```python
from build123d import *

# Parameters (mm, degrees)
CORTE_EXTRUS_O3_REACH         = 46.677
RESSALTO_EXTRUS_O1_DEPTH      = 2
RESSALTO_EXTRUS_O1_DEPTH_BACK = 7.7
ESBO_O4_R                     = 7.5
ESBO_O4_R_2                   = 3.25


# Read off the part's stored shape, not the designer's step: PadrãoCircular1
with BuildPart() as part:
    # Esboço1 → Revolução1 (revolve)
    with BuildSketch(Plane.XY, mode=Mode.PRIVATE) as revolu_o1_sk:
        Polygon((3.25, 14), (3.25, 11.5), (5, 11.5), (5, 6.3), (15, 6.3), (15, 9), (30, 9), (30, 14), align=None)
    revolve(revolu_o1_sk.sketch.rotate(Axis((0, 0, 0), (0, 1, 0)), 90), axis=Axis((0, 0, 0), (0, 1, 0)))

    # Esboço2 → Corte-extrusão3 (cut, up to next)
    with BuildSketch(Plane(origin=(0, 0, 0), x_dir=(1, 0, 0), z_dir=(0, 1, 0)), mode=Mode.PRIVATE) as corte_extrus_o3_sk1:
        with BuildLine():
            ThreePointArc((2.923717047, 9.56304756), (1.478094111, 9.890158634), (0, 10))
            ThreePointArc((0, 10), (-1.5, 11.5), (0, 13))
            ThreePointArc((0, 13), (1.921522345, 12.857206224), (3.800832161, 12.431961828))
            ThreePointArc((3.800832161, 12.431961828), (4.796731738, 10.558947136), (2.923717047, 9.56304756))
        make_face()
    corte_extrus_o3_tool1 = extrude(corte_extrus_o3_sk1.sketch, amount=CORTE_EXTRUS_O3_REACH, mode=Mode.PRIVATE) & part.part
    add(corte_extrus_o3_tool1.solids().sort_by_distance((1.688498, 0, -11.298001))[0], mode=Mode.SUBTRACT)

    # Esboço4 → Ressalto-extrusão1 (add, two sides: drawn at the far end of the back side and taken through both)
    with BuildSketch(Plane(origin=(0, 14, 0), x_dir=(1, 0, 0), z_dir=(0, 1, 0)).offset(-RESSALTO_EXTRUS_O1_DEPTH_BACK)):
        with Locations(Location((0, 0, 0), (0, 0, 270))):
            Circle(ESBO_O4_R)
        with Locations(Location((0, 0, 0), (0, 0, 270))):
            Circle(ESBO_O4_R_2, mode=Mode.SUBTRACT)
    extrude(amount=RESSALTO_EXTRUS_O1_DEPTH + RESSALTO_EXTRUS_O1_DEPTH_BACK)

    # Esboço10 → Escareado para parafuso de máquina com cabeça chata de M21 (revolve, cut)
    with BuildSketch(Plane(origin=(0, 14, -22.5), x_dir=(0, 0, 1), z_dir=(1, 0, 0))):
        Polygon((0, 0), (0, 5.660946681), (1.1, 5), (1.1, 1.1), (2.2, 0), align=None)
    revolve(axis=Axis((0, 20.35, -22.5), (0, -1, 0)), mode=Mode.SUBTRACT)

    # PadrãoCircular1 outline → PadrãoCircular1 (revolve, cut)
    with BuildSketch(Plane(origin=(22.5, 0, 0), x_dir=(1, 0, 0), z_dir=(0, 0, 1))):
        Polygon((0, 9), (1.1, 9), (1.1, 12.9), (2.2, 14), (0, 14), align=None)
    revolve(axis=Axis((22.5, 0, 0), (0, 1, 0)), mode=Mode.SUBTRACT)

    # Padr_oCircular1 2 outline → Padr_oCircular1 2 (revolve, cut)
    with BuildSketch(Plane.XY.offset(22.5)):
        Polygon((0, 9), (1.1, 9), (1.1, 12.9), (2.2, 14), (0, 14), align=None)
    revolve(axis=Axis((0, 0, 22.5), (0, 1, 0)), mode=Mode.SUBTRACT)

    # Padr_oCircular1 3 outline → Padr_oCircular1 3 (revolve, cut)
    with BuildSketch(Plane(origin=(-22.5, 0, 0), x_dir=(1, 0, 0), z_dir=(0, 0, 1))):
        Polygon((0, 9), (1.1, 9), (1.1, 12.9), (2.2, 14), (0, 14), align=None)
    revolve(axis=Axis((-22.5, 0, 0), (0, 1, 0)), mode=Mode.SUBTRACT)


solid = part.part
```
Source: CAD feature listing. Evaluate the final solid. Frame: model axes, mm. A direction names the side the tool comes from. Round coordinates to 2 decimals unless told otherwise and drop trailing zeros. Order: outer loops, then holes, each group sorted by start corner. A loop starts at its lowest first (then second) coordinate and runs counter-clockwise, first axis right, second up. Notation, with made-up numbers: (10.25, 63) -> (33.25, 63) arc R18 ccw to (33.25, 89) -> close; hole circle Ø10 at (54.25, 19.25). An arc over 180 degrees is marked (long way). One line per item, written item: value. Start each with the question number.
Q1. Section query B-B (y = 10). Return the cut outline in (x, z), plus the area to 3 significant figures.
Q2. Section query D-D (z = -11.5). Return the cut outline in (x, y).
Q3. Draft query along Z for faces 4 (the cylindrical face through (21.4, 11, 0)), 5 (the cylindrical face through (0.33, 14.986, -7.493)), 6 (the flat face through (-2, 16, 3)). Return one class per face: pulls with the +Z half, pulls with the -Z half, needs draft (parallel to the pull), parting line crosses it, or undercut.
Q4. Access query for faces 1 (the cylindrical face through (-12.65, 7.67, -8.06)), 2 (the cylindrical face through (-1.5, 10.1, -11.5)), 3 (the flat face through (6, 14, -6)). Directions: +Z, -Z, +X, -X, +Y, -Y. A direction counts if a zero-diameter tool reaches every point of the face in a straight line with its end or side. Return the directions, or none.
Q5. Section query C-C (z = 0). Return the cut outline in (x, y), plus the area to 3 significant figures.
Q6. Material intervals for probe 1 along X at (y, z) = (10.5, 0); probe 2 along Y at (x, z) = (27, -2.5); probe 3 along X at (y, z) = (13.5, -18.5), sorted ascending.
Q7. Section query A-A (x = 22.5). Return the cut outline in (y, z), plus the area to 3 significant figures.
Q8. Pin query (flat end, axial travel): pin 1 (5 mm diameter, centred on y = 9, z = -11.5, fed in from +X); pin 2 (2 mm diameter, centred on x = -3.5, y = 8.5, fed in from +Z); pin 3 (3 mm diameter, centred on x = 0, z = 22.5, fed in from +Y). Return the tip coordinate at first contact, or that it passes through.
Findings below:
1. outline: circle Ø60 at (0, 0); hole circle Ø2.2 at (-22.5, 0); hole circle Ø6.5 at (0, 0); hole circle Ø2.2 at (0, -22.5); hole circle Ø2.2 at (0, 22.5); hole (0, -13) arc R13 ccw to (3.8, -12.43) arc R1.5 ccw to (2.92, -9.56) arc R10 cw to (0, -10) arc R1.5 ccw to start; hole circle Ø2.2 at (22.5, 0)
1. area: 2,760 mm²
2. outline: (-27.71, 9) -> (-9.63, 9) -> (-9.63, 6.3) -> (-1.5, 6.3) -> (-1.5, 14) -> (-27.71, 14) -> close; (4.78, 6.3) -> (9.63, 6.3) -> (9.63, 9) -> (27.71, 9) -> (27.71, 14) -> (4.78, 14) -> close
3. face 4: undercut
3. face 5: parting line crosses it
3. face 6: needs draft
4. face 1: -Y
4. face 2: +Y, -Y
4. face 3: +Y
5. outline: (-30, 9) -> (-23.6, 9) -> (-23.6, 12.9) -> (-24.7, 14) -> (-30, 14) -> close; (-21.4, 9) -> (-15, 9) -> (-15, 6.3) -> (-3.25, 6.3) -> (-3.25, 16) -> (-7.5, 16) -> (-7.5, 14) -> (-20.3, 14) -> (-21.4, 12.9) -> close; (3.25, 6.3) -> (15, 6.3) -> (15, 9) -> (21.4, 9) -> (21.4, 12.9) -> (20.3, 14) -> (7.5, 14) -> (7.5, 16) -> (3.25, 16) -> close; (23.6, 9) -> (30, 9) -> (30, 14) -> (24.7, 14) -> (23.6, 12.9) -> close
5. area: 324 mm²
6. probe 1: -30 to -23.6, -21.4 to -3.25, 3.25 to 21.4, 23.6 to 30
6. probe 2: 9 to 14
6. probe 3: -23.62 to 23.62
7. outline: (9, -19.84) -> (14, -19.84) -> (14, -2.2) -> (12.9, -1.1) -> (9, -1.1) -> close; (9, 1.1) -> (12.9, 1.1) -> (14, 2.2) -> (14, 19.84) -> (9, 19.84) -> close
7. area: 186 mm²
8. pin 1: x = 28.62
8. pin 2: z = 29.88
8. pin 3: y = 13.3
